Can you work these out from the drawing? Everything is in mm from the part's minimum corner. Coordinates: 2 decimals unless noted, no trailing zeros. Loops run counter-clockwise (first coordinate to the right, second up) from the corner with the lowest first, then second, coordinate; pieces in that order, holes last. Notation, with made-up numbers: M 38,78 L 60,78 A17 cw 60,111 Z; hole C 28.5,-1.75 d2. An arc over 180 degrees is marked long. Write each question's results on one line, items separated by ' | '.
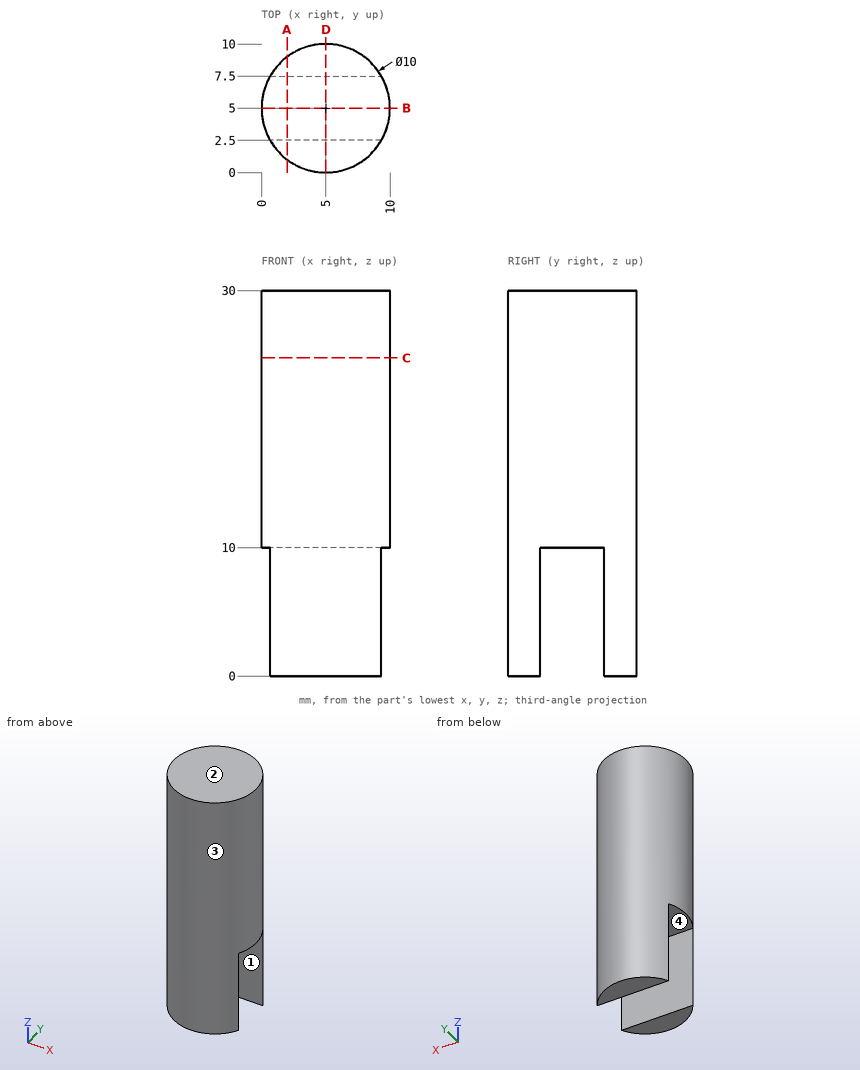
(1) Imagine slicing it at D-D, the plane x = 5. List the corners of the cut face in (y, z) for me.
Reported:
outline: M 0,0 L 2.5,0 L 2.5,10 L 7.5,10 L 7.5,0 L 10,0 L 10,30 L 0,30 Z
(2) Imagine slicing it at C-C, the plane z = 24.75. List the corners of the cut face in (x, y) for me.
Reported:
outline: C 5,5 d10
(3) Imagine slicing it at A-A, the plane x = 2. List the corners of the cut face in (y, z) for me, and give its area (3 significant figures).
Reported:
outline: M 1,0 L 2.5,0 L 2.5,10 L 7.5,10 L 7.5,0 L 9,0 L 9,30 L 1,30 Z | area: 190 mm2
(4) Imagine slicing it at B-B, the plane y = 5. List the corners of the cut face in (x, z) for me.
Reported:
outline: M 0,10 L 10,10 L 10,30 L 0,30 Z
(5) Will these pins go through, and if not, where does the flat tip stop? P1, Ø4, axis at x = 3, y = 5, coming from the -Z side; P2, Ø1.5, axis at y = 7, z = 11, coming from the -X side.
Reported:
P1: stops at z = 10 | P2: stops at x = 0.16
(6) If we mould it in two halves opening along Y, with no side actions, what happens to the marked faces 1, 2, 3 and 4? For each: released by +Y, released by -Y, zero draft, split by the parting line, or undercut.
Reported:
face 1: undercut | face 2: zero draft | face 3: split by the parting line | face 4: undercut
(7) Please list where these lines run through material, in increasing order: probe 1 along Y at (x, z) = (2.5, 2.25); probe 2 along Z at (x, y) = (7.75, 4); probe 3 along Y at (x, z) = (2.75, 4). Write a range as from..to.
Reported:
probe 1: y = 0.67..2.5, 7.5..9.33 | probe 2: z = 10..30 | probe 3: y = 0.53..2.5, 7.5..9.47
